Work out the finished part from the listing and answer in its coordinate system (mm). A direction names the side the tool comes from. Round coordinates to 2 decimals unless told otherwise and drop trailing zeros. Loops run counter-clockwise (first coordinate to the right, second up) from the corner with the lowest first, then second, coordinate; pieces in that order, holes last. Notation, with made-up numbers: (89.5, 11.25) - (95.5, 11.25) arc R28 cw to (95.5, 40.25) - close; hole circle Ø5 at (-32, -3.75). An arc over 180 degrees is marked (long way). Answer as CSV lines item,"result". Start each with the question number.
Q1. For faces 4 (the face through (28, 20, -18)), 5 (the face through (0, 2, 0)), 6 (the face through (-7.6, 15, 33.5)), determine the directions among +Z, -Z, +X, -X, +Y, -Y from which every point of the face is accessible in a straight line to the end or side of a thin tool.
Q2. Straight lines are drawn through the part: L1, parallel to Z at x = 0, y = 8.25; L2, parallel to Z at x = 0, y = 15.5. For each, find the intervals that lie inside material, in ascending order. Write a range as [from, to].
Q3. The mould has two halves that part along X. Classify faces 1 (the face through (0, 0, 0)), 2 (the face through (28, 8, 21)), 3 (the face through (-30.5, 11.4, 12.6)): +X half, -X half, draft (parallel to the pull), parting line (faces both ways), or undercut.
Q4. Each of these flat-tipped pins is pushed along its axis until it touches: pin 1 Ø5 at (y, z) = (14, 4) entering from +X; pin 2 Ø1 at (x, y) = (-6, 13) entering from +Z; pin 3 Ø1 at (x, y) = (-6.5, 11) entering from -Z. Where does it stop, or does it pass through?
Q5. Section A-A on y = 4.5 is taken. Write down the section's boundary in (x, z).
```python
from build123d import *

# Parameters (mm, degrees)
CHAMFER_1_SIZE = 1
THREAD_1_PITCH = 2
FILLET_1_R     = 1


with BuildPart() as part:
    # Sketch 1 → Повернуть1 (revolve)
    with BuildSketch(Plane.XY):
        Polygon((0, 0), (-35, 0), (-35, 15), (-34, 15), (-34, 20), (-33, 20), (-33, 2), (0, 2), align=None)
    revolve(axis=Axis((0, 2, 0), (0, -1, 0)))

    # Фаска1
    chamfer_1_edges = [part.edges().sort_by_distance(p)[0] for p in [
        (35, 0, 0),
    ]]
    chamfer(chamfer_1_edges, length=CHAMFER_1_SIZE)

    # Резьба1: the profile of Sketch 1 2 profile screwed along a right-hand helix of 2.5 turns, 10 arcs to a turn; built about Z, then put on its axis
    thread_1_z = Axis((0, 0, 0), (0, 0, 1))
    thread_1_corners = [(33.9997, 0, -0.000173205), (34.687407661, 0, 0.396874998), (34.687407661, 0, 0.555624998), (33.9997, 0, 0.952673202)]
    with BuildLine(mode=Mode.PRIVATE) as thread_1_profile:
        Line(thread_1_corners[0], thread_1_corners[1])
        Line(thread_1_corners[1], thread_1_corners[2])
        Line(thread_1_corners[2], thread_1_corners[3])
        Line(thread_1_corners[3], thread_1_corners[0])
    thread_1_cap = Face(thread_1_profile.wire())
    thread_1_turn_angles = [0, 18, 36, 54, 72, 90, 108, 126, 144, 162, 180, 198, 216, 234, 252, 270, 288, 306, 324, 342, 360]
    thread_1_turn_weights = [1, 0.9510565162951535, 1, 0.9510565162951535, 1, 0.9510565162951535, 1, 0.9510565162951535, 1, 0.9510565162951535, 1, 0.9510565162951535, 1, 0.9510565162951535, 1, 0.9510565162951535, 1, 0.9510565162951535, 1, 0.9510565162951535, 1]
    thread_1_turn_rails = [Edge.make_bspline([Vector(p[0], p[1], 0).rotate(thread_1_z, thread_1_turn_angles[k]) / thread_1_turn_weights[k] + Vector(0, 0, p[2] + THREAD_1_PITCH * thread_1_turn_angles[k] / 360) for k in range(21)], [0, 0, 0, 1, 1, 2, 2, 3, 3, 4, 4, 5, 5, 6, 6, 7, 7, 8, 8, 9, 9, 10, 10, 10], 2, thread_1_turn_weights) for p in thread_1_corners]
    thread_1_turn_sides = [Face.make_surface_from_curves(thread_1_turn_rails[p[0]], thread_1_turn_rails[p[1]]) for p in [(0, 1), (1, 2), (2, 3), (3, 0)]]
    thread_1_last_angles = [720, 738, 756, 774, 792, 810, 828, 846, 864, 882, 900]
    thread_1_last_weights = [1, 0.9510565162951535, 1, 0.9510565162951535, 1, 0.9510565162951535, 1, 0.9510565162951535, 1, 0.9510565162951535, 1]
    thread_1_last_rails = [Edge.make_bspline([Vector(p[0], p[1], 0).rotate(thread_1_z, thread_1_last_angles[k]) / thread_1_last_weights[k] + Vector(0, 0, p[2] + THREAD_1_PITCH * thread_1_last_angles[k] / 360) for k in range(11)], [0, 0, 0, 1, 1, 2, 2, 3, 3, 4, 4, 5, 5, 5], 2, thread_1_last_weights) for p in thread_1_corners]
    thread_1_last_sides = [Face.make_surface_from_curves(thread_1_last_rails[p[0]], thread_1_last_rails[p[1]]) for p in [(0, 1), (1, 2), (2, 3), (3, 0)]]
    thread_1 = Plane(origin=(0, 20, 0), x_dir=(-1, 0, 0), z_dir=(0, -1, 0)) * Solid(Shell([*[p.moved(Location((0, 0, THREAD_1_PITCH * i))) for i in range(2) for p in thread_1_turn_sides], *thread_1_last_sides, thread_1_cap, thread_1_cap.rotate(thread_1_z, 900).moved(Location((0, 0, THREAD_1_PITCH * 900 / 360)))]))
    add(thread_1)

    # Скругление1
    fillet_1_edges = [part.edges().sort_by_distance(p)[0] for p in [
        (33, 2, 0),
    ]]
    fillet(fillet_1_edges, radius=FILLET_1_R)


solid = part.part
```
Findings:
1,face 4,"+Z, -Z, +X, -X, +Y"
1,face 5,"+Y"
1,face 6,"none"
2,L1,"z = [-35, -33], [33, 35]"
2,L2,"z = [-34, -33], [33, 34]"
3,face 1,"draft"
3,face 2,"parting line"
3,face 3,"undercut"
4,pin 1,"stops at x = 34.97"
4,pin 2,"stops at z = 34.57"
4,pin 3,"stops at z = -34.48"
5,outline,"circle Ø70 at (0, 0); hole circle Ø66 at (0, 0)"
